Here's how the part is built. I have some questions about the finished solid (model axes, mm). Face numbers are marked on the shaded views. A direction names the side the tool comes from. Coordinates: 2 decimals unless noted, no trailing zeros. Order: outer loops, then holes, each group sorted by start corner. A loop starts at its lowest first (then second) coordinate and runs counter-clockwise, first axis right, second up. Notation, with made-up numbers: (-21.75, -32) - (37.25, -32) arc R32 ccw to (37.25, 4) - close; hole circle Ø3 at (77, 8). An arc over 180 degrees is marked (long way). Answer as CSV lines item,"result". Start each with the question number.
Item 1: Imagine slicing it at B-B on x = 0. List the corners of the cut face in (y, z) for me (1 decimal).
Item 2: I need wall thicknesses on line 1 (Z direction, x = -312, y = 55.5); line 2 (X direction, y = 31.5, z = -45.5); line 3 (Z direction, x = -308, y = 23). Which ranges of each line are inside material? Lowest first, please.
Item 3: I'm going to push flat-ended pins straight in: pin 1 (8 mm diameter, centred on x = 211.5, y = 27, fed in from +Z); pin 2 (6 mm diameter, centred on x = -259.5, y = 27.5, fed in from +Z); pin 3 (2 mm diameter, centred on x = -163.5, y = 109.5, fed in from -Z). Where does each tip first touch, or does it pass through?
Item 4: Imagine slicing it at C-C on y = 18.5. Count the separate pieces of the cut face and the enclosed holes in it, and give its area (3 significant figures).
Item 5: Imagine slicing it at A-A on z = 0. List the corners of the cut face in (x, y) for me (1 decimal), and give its area (3 significant figures).
Item 6: On a 3-axis mill with a long thin cutter (end or side, diameter ignored), from which of +Z, -Z, +X, -X, +Y, -Y can I reach the whole of each face in a straight line? I mean the marked faces 4 and 5. Say none if no direction works.
Item 7: Imagine slicing it at D-D on y = 116.5. List the corners of the cut face in (x, z) for me (3 decimals).
Item 8: We'd pull the mould along X, two halves only. Please class the marked faces 1, 2 and 3: pulls with the +X half, pulls with the -X half, needs draft (parallel to the pull), parting line crosses it, or undercut.
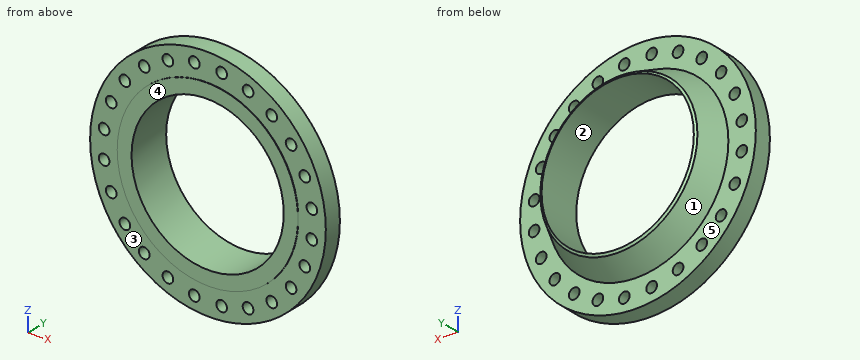
Autodesk Inventor part; units mm, degrees
ref_plane "YZ Plane" through (0, 0, 0) normal (1, 0, 0) x (0, 1, 0)
ref_plane "XZ Plane" through (0, 0, 0) normal (0, 1, 0) x (-1, 0, 0)
ref_plane "XY Plane" through (0, 0, 0) normal (0, 0, 1) x (1, 0, 0)
sketch "Sketch1" plane through (0, 0, 0) normal (0, 0, 1) x (1, 0, 0)
  line L0 (0, 0) -> (0, 168.2115) construction
  line L1 (-295.275, 168.2115) -> (-295.275, 0)
  line L2 (-295.275, 0) -> (-350.774, 0)
  line L3 (-350.774, 0) -> (-350.774, 1.5875)
  line L4 (-350.774, 1.5875) -> (-457.2, 1.5875)
  line L5 (-457.2, 1.5875) -> (-457.2, 69.9135)
  line L6 (-457.2, 69.9135) -> (-350.774, 69.9135)
  line L7 (-350.774, 69.9135) -> (-304.8, 162.7122)
  line L8 (-304.8, 162.7122) -> (-295.275, 168.2115)
  line L9 (-406.4, 69.9135) -> (-406.4, 1.5875) construction
  dimension "WB" = 590.55
  dimension "d1" = 1.5875
  dimension "WL" = 166.624
  dimension "Thickness" = 68.326
  dimension "R" = 701.548
  dimension "OD" = 914.4
  dimension "HB" = 701.548
  dimension "HT" = 609.6
  dimension "d8" = 60
  dimension "BC" = 812.8
revolve "Revolution1" add sketch "Sketch1" angle 360 about axis through (0, 0, 0) along (0, 1, 0)
sketch "Sketch2" plane through (0, 69.9135, 0) normal (0, 1, 0) x (1, 0, 0)
  line L0 (0, 0) -> (0, 457.2) construction
  circle A0 centre (0, 0) radius 457.2
  line L1 (0, 0) -> (53.0458, 402.9232) construction
  dimension "d11" = 7.5
  dimension "d12" = 406.4
hole "Hole1" at (53.0458, 69.9135, -402.9232) direction (0, -1, 0) diameter 41.402 depth 68.326
pattern_circular "Circular Pattern1" count 24 over 360 about axis through (0, -10, 0) along (0, 1, 0) of "Hole1"
equation "\"d12\" = 0.5 * BC"
properties part number "ANSI-B300-24W"
Responses:
1,outline,"(0, -350.8) - (1.6, -350.8) - (1.6, -457.2) - (69.9, -457.2) - (69.9, -350.8) - (162.7, -304.8) - (168.2, -295.3) - (0, -295.3) - close; (0, 295.3) - (168.2, 295.3) - (162.7, 304.8) - (69.9, 350.8) - (69.9, 457.2) - (1.6, 457.2) - (1.6, 350.8) - (0, 350.8) - close"
2,line 1,"z = -334.2 to -265.29, -229.51 to 229.51, 265.29 to 334.2"
2,line 2,"x = -454.93 to -422.2, -383.65 to -291.75, 291.75 to 383.65, 422.2 to 454.93"
2,line 3,"z = -337.89 to -262.25, -232.55 to 232.55, 262.25 to 337.89"
3,pin 1,"stops at z = 407.4"
3,pin 2,"stops at z = 378.47"
3,pin 3,"stops at z = -288.79"
4,separate pieces,"1"
4,enclosed holes,"25"
4,area,"350,000 mm^2"
5,outline,"(-457.2, 1.6) - (-350.8, 1.6) - (-350.8, 0) - (-295.3, 0) - (-295.3, 168.2) - (-304.8, 162.7) - (-350.8, 69.9) - (-457.2, 69.9) - close; (295.3, 0) - (350.8, 0) - (350.8, 1.6) - (457.2, 1.6) - (457.2, 69.9) - (350.8, 69.9) - (304.8, 162.7) - (295.3, 168.2) - close"
5,area,"28,400 mm^2"
6,face 4,"+Z, -Z, +X, -X, -Y"
6,face 5,"+Y"
7,outline,"circle Ø655.389 at (0, 0); hole circle Ø590.55 at (0, 0)"
8,face 1,"parting line crosses it"
8,face 2,"undercut"
8,face 3,"needs draft"
